The listing builds one solid part. Answer for the finished solid, in the listing's coordinates (mm). Coordinates: 2 decimals unless noted, no trailing zeros. Order: outer loops, then holes, each group sorted by start corner. A loop starts at its lowest first (then second) coordinate and runs counter-clockwise, first axis right, second up. Notation, with made-up numbers: (45.25, -36.5) - (66.25, -36.5) arc R23 ccw to (66.25, -14.5) - close; hole circle Ø11 at (5, 38.5). An arc over 180 degrees is marked (long way). Use one line per item in the form item = value. Start each with the question number.
Item 1: Consider line 1 along Z through (x, y) = (0, 1.85); line 2 along X through (y, z) = (0.35, -1.5); line 3 along Z through (x, y) = (0.5, 2.55). Determine where each line is inside the solid, lowest interval first. Write a range as [from, to].
Item 2: Section C-C, the plane y = 2.6 is taken. Write down the section's boundary in (x, z) (3 decimals).
Item 3: Section D-D, the plane x = 16.5 is taken. Write down the section's boundary in (y, z) (3 decimals), and give its area (3 significant figures).
Item 4: Section B-B, the plane z = 0 is taken. Write down the section's boundary in (x, y) (3 decimals).
Item 5: Section A-A, the plane x = 0 is taken. Write down the section's boundary in (y, z) (3 decimals).
from build123d import *

# Parameters (mm, degrees)
SKETCH1_R           = 59.309
SKETCH1_R_2         = 51.181
BOSS_EXTRUDE1_DEPTH = 3.175
SKETCH2_R           = 2.159
CUT_EXTRUDE1_DEPTH  = 3.175
CIRPATTERN1_COUNT   = 6


with BuildPart() as part:
    # Sketch1 → Boss-Extrude1 (new body)
    with BuildSketch(Plane(origin=(0, 0, 0), x_dir=(1, 0, 0), z_dir=(0, 1, 0))):
        Circle(SKETCH1_R)
        Circle(SKETCH1_R_2, mode=Mode.SUBTRACT)
    extrude(amount=BOSS_EXTRUDE1_DEPTH)

    # Sketch2 → Cut-Extrude1 (cut)
    with BuildSketch(Plane(origin=(0, 3.175, 0), x_dir=(1, 0, 0), z_dir=(0, 1, 0))):
        with Locations((0, 54.61)):
            Circle(SKETCH2_R)
    cut_extrude1 = extrude(amount=-CUT_EXTRUDE1_DEPTH, mode=Mode.SUBTRACT)

    # CirPattern1: Cut-Extrude1 ×6 about axis
    cirpattern1_axis = Axis((0, 0, 0), (0, 1, 0))
    for i in range(1, CIRPATTERN1_COUNT):
        add(cut_extrude1.rotate(cirpattern1_axis, i * 360 / CIRPATTERN1_COUNT), mode=Mode.SUBTRACT)


solid = part.part
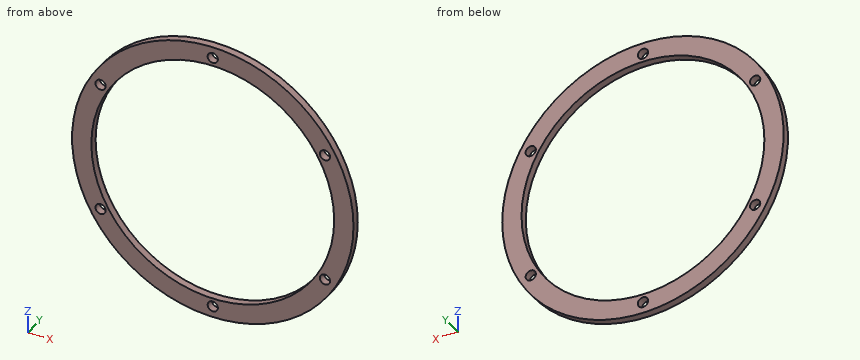
Response:
q1.line_1 = [-59.31, -56.77], [-52.45, -51.18], [51.18, 52.45], [56.77, 59.31]
q1.line_2 = [-59.29, -51.16], [51.16, 59.29]
q1.line_3 = [-59.31, -56.71], [-52.51, -51.18], [51.18, 52.51], [56.71, 59.31]
q2.outline = circle Ø118.618 at (0, 0); hole circle Ø102.362 at (0, 0); hole circle Ø4.318 at (-47.294, -27.305); hole circle Ø4.318 at (-47.294, 27.305); hole circle Ø4.318 at (0, -54.61); hole circle Ø4.318 at (0, 54.61); hole circle Ø4.318 at (47.294, -27.305); hole circle Ø4.318 at (47.294, 27.305)
q3.outline = (0, -56.968) - (3.175, -56.968) - (3.175, -48.448) - (0, -48.448) - close; (0, 48.448) - (3.175, 48.448) - (3.175, 56.968) - (0, 56.968) - close
q3.area = 54.1 mm2
q4.outline = (-59.309, 0) - (-51.181, 0) - (-51.181, 3.175) - (-59.309, 3.175) - close; (51.181, 0) - (59.309, 0) - (59.309, 3.175) - (51.181, 3.175) - close
q5.outline = (0, -59.309) - (3.175, -59.309) - (3.175, -56.769) - (0, -56.769) - close; (0, -52.451) - (3.175, -52.451) - (3.175, -51.181) - (0, -51.181) - close; (0, 51.181) - (3.175, 51.181) - (3.175, 52.451) - (0, 52.451) - close; (0, 56.769) - (3.175, 56.769) - (3.175, 59.309) - (0, 59.309) - close
